```python
from build123d import *

# Parameters (mm, degrees)
SKETCH_1_R          = 12.5
EXTRUDE_1_DEPTH     = 27
CUT_EXTRUDE_START   = -37
CUT_EXTRUDE_1_DEPTH = 37
CUT_EXTRUDE_START_2 = 10
CUT_EXTRUDE_2_DEPTH = 43
SKETCH_4_W          = 14
SKETCH_4_H          = 25
CUT_EXTRUDE_3_DEPTH = 30
FILLET_1_R          = 4
SKETCH_7_R          = 4
SKETCH_5_R          = 4
CUT_EXTRUDE_4_DEPTH = 34
SKETCH_9_W          = 2.5
SKETCH_9_H          = 6
CUT_EXTRUDE_5_DEPTH = 34
SKETCH_10_R         = 1.5
CUT_EXTRUDE_6_DEPTH = 34
FILLET_3_R          = 1.5
SKETCH_11_R         = 2.5
EXTRUDE_2_DEPTH     = 14.5
SKETCH_12_R         = 2
EXTRUDE_3_DEPTH     = 10
FILLET_4_R          = 10


with BuildPart() as part:
    # 草图1 → 凸台-拉伸1 (new body)
    with BuildSketch(Plane(origin=(0, 0, 0), x_dir=(1, 0, 0), z_dir=(0, 1, 0))):
        with Locations(Location((0, 0, 0), (0, 0, 270))):
            Circle(SKETCH_1_R)
    extrude(amount=-EXTRUDE_1_DEPTH)

    # 草图2 → 切除-拉伸1 (cut)
    with BuildSketch(Plane(origin=(0, -27, 0), x_dir=(-1, 0, 0), z_dir=(0, -1, 0)).offset(CUT_EXTRUDE_START)):
        with BuildLine():
            Line((-10, 7.5), (10, 7.5))
            ThreePointArc((10, 7.5), (0, 12.5), (-10, 7.5))
        make_face()
        with BuildLine():
            Line((-10, -7.5), (10, -7.5))
            ThreePointArc((10, -7.5), (0, -12.5), (-10, -7.5))
        make_face()
    extrude(amount=CUT_EXTRUDE_1_DEPTH, mode=Mode.SUBTRACT)

    # 草图3 → 切除-拉伸2 (cut)
    with BuildSketch(Plane(origin=(0, 0, 0), x_dir=(1, 0, 0), z_dir=(0, 1, 0)).offset(CUT_EXTRUDE_START_2)):
        with BuildLine():
            Line((-12, 3.5), (-12, -3.5))
            ThreePointArc((-12, -3.5), (-12.5, 0), (-12, 3.5))
        make_face()
        with BuildLine():
            Line((12, 3.5), (12, -3.5))
            ThreePointArc((12, -3.5), (12.5, 0), (12, 3.5))
        make_face()
    extrude(amount=-CUT_EXTRUDE_2_DEPTH, mode=Mode.SUBTRACT)

    # 草图4 → 切除-拉伸3 (cut)
    with BuildSketch(Plane.XY.offset(7.5)):
        with Locations((0, -14.5)):
            Rectangle(SKETCH_4_W, SKETCH_4_H)
    extrude(amount=-CUT_EXTRUDE_3_DEPTH, mode=Mode.SUBTRACT)

    # 圆角1
    fillet_1_edges = [part.edges().sort_by_distance(p)[0] for p in [
        (-7, -2, 0),
        (7, -2, 0),
    ]]
    fillet(fillet_1_edges, radius=FILLET_1_R)

    # 草图7 → 放样2 section 0
    with BuildSketch(Plane(origin=(0, 0, 0), x_dir=(1, 0, 0), z_dir=(0, 1, 0))):
        Circle(SKETCH_7_R)
    # 草图5 → 放样2 section 1
    with BuildSketch(Plane(origin=(0, 1, 0), x_dir=(1, 0, 0), z_dir=(0, 1, 0))):
        Circle(SKETCH_5_R)
    loft()

    # 草图8 → 切除-拉伸4 (cut)
    with BuildSketch(Plane.ZY.offset(12)):
        with BuildLine():
            Line((-2, -27), (2, -27))
            Line((2, -27), (2, -20.464101615))
            ThreePointArc((2, -20.464101615), (0, -13), (-2, -20.464101615))
            Line((-2, -20.464101615), (-2, -27))
        make_face()
    extrude(amount=-CUT_EXTRUDE_4_DEPTH, mode=Mode.SUBTRACT)

    # 草图9 → 切除-拉伸5 (cut)
    with BuildSketch(Plane.ZY.offset(12)):
        with Locations((6.25, -24)):
            Rectangle(SKETCH_9_W, SKETCH_9_H)
        with Locations((-6.25, -24)):
            Rectangle(SKETCH_9_W, SKETCH_9_H)
    extrude(amount=-CUT_EXTRUDE_5_DEPTH, mode=Mode.SUBTRACT)

    # 草图10 → 切除-拉伸6 (cut)
    with BuildSketch(Plane.XY.offset(5)):
        with Locations(Location((-9.5, -24.5, 0), (0, 0, 270))):
            Circle(SKETCH_10_R)
        with Locations(Location((9.5, -24.5, 0), (0, 0, 270))):
            Circle(SKETCH_10_R)
    extrude(amount=-CUT_EXTRUDE_6_DEPTH, mode=Mode.SUBTRACT)

    # 圆角3
    fillet_3_edges = [part.edges().sort_by_distance(p)[0] for p in [
        (-12, -27, 2.75),
        (-12, -27, -2.75),
        (-7, -27, -3.5),
        (-7, -27, 3.5),
        (7, -27, -3.5),
        (7, -27, 3.5),
        (12, -27, 2.75),
        (12, -27, -2.75),
    ]]
    fillet(fillet_3_edges, radius=FILLET_3_R)

    # 草图11 → 凸台-拉伸2 (add)
    with BuildSketch(Plane(origin=(0, 1, 0), x_dir=(1, 0, 0), z_dir=(0, 1, 0))):
        with Locations(Location((0, 0, 0), (0, 0, 90))):
            Circle(SKETCH_11_R)
    extrude(amount=EXTRUDE_2_DEPTH)

    # 草图12 → 凸台-拉伸3 (add)
    with BuildSketch(Plane(origin=(0, 15.5, 0), x_dir=(1, 0, 0), z_dir=(0, 1, 0))):
        with Locations(Location((0, 0, 0), (0, 0, 270))):
            Circle(SKETCH_12_R)
    extrude(amount=EXTRUDE_3_DEPTH)

    # 圆角4
    # the kernel refuses this fillet: 10 mm, written as the material it takes off along each edge
    with BuildSketch(Plane(origin=(-9.535945694, -21, 7.5), x_dir=(0, 1, 0), z_dir=(1, 0, 0)), Plane(origin=(-26.535945694, -21, 7.5), x_dir=(0, 1, 0), z_dir=(1, 0, 0))) as fillet_4_piece_1:
        with BuildLine():
            CenterArc((6.614378278, -10), FILLET_4_R, 90, 41.409622109)
            Line((0, -2.5), (-0.132287566, -2.35))
            ThreePointArc((-0.132287566, -2.35), (-0.2, -1.25), (-0.2, 0))
            Line((-0.2, 0), (0, 0.2))
            Line((0, 0.2), (6.614378278, 0.2))
            Line((6.614378278, 0.2), (6.614378278, 0))
        make_face()
    extrude(amount=36.071891388, mode=Mode.SUBTRACT)
    with BuildSketch(Plane(origin=(-9.535945694, -21, -7.5), x_dir=(0, 0, 1), z_dir=(1, 0, 0))) as fillet_4_piece_2:
        with BuildLine():
            CenterArc((10, -6.614378278), FILLET_4_R, 138.590377891, 41.409622109)
            Line((0, -6.614378278), (-0.2, -6.614378278))
            Line((-0.2, -6.614378278), (-0.2, 0))
            Line((-0.2, 0), (0, 0.2))
            ThreePointArc((0, 0.2), (1.25, 0.2), (2.35, 0.132287566))
            Line((2.35, 0.132287566), (2.5, 0))
        make_face()
    extrude(amount=36.071891388, mode=Mode.SUBTRACT)
    with BuildSketch(Plane(origin=(-26.535945694, -21, -7.5), x_dir=(0, 1, 0), z_dir=(1, 0, 0))) as fillet_4_piece_3:
        with BuildLine():
            CenterArc((6.614378278, 10), FILLET_4_R, 228.590377891, 41.409622109)
            Line((0, 2.5), (-0.132287566, 2.35))
            ThreePointArc((-0.132287566, 2.35), (-0.2, 1.25), (-0.2, 0))
            Line((-0.2, 0), (0, -0.2))
            Line((0, -0.2), (6.614378278, -0.2))
            Line((6.614378278, -0.2), (6.614378278, 0))
        make_face()
    extrude(amount=36.071891388, mode=Mode.SUBTRACT)


solid = part.part
```
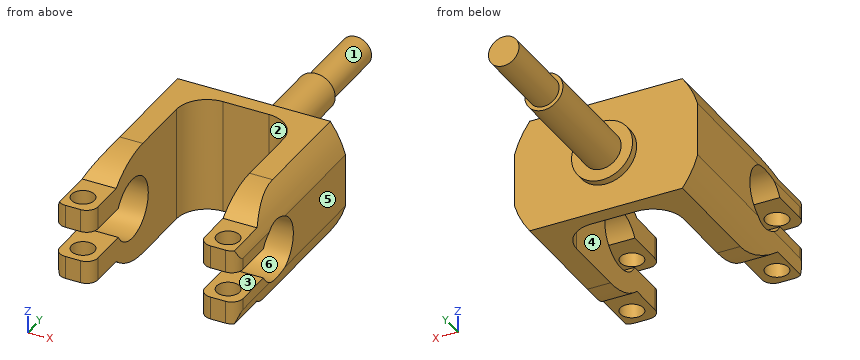
Design review of the part built by this model. Coordinates are the model's own, in mm. Face numbers are marked on the shaded views. A direction names the side the tool comes from. Coordinates: 2 decimals unless noted, no trailing zeros. Order: outer loops, then holes, each group sorted by start corner. A loop starts at its lowest first (then second) coordinate and runs counter-clockwise, first axis right, second up. Notation, with made-up numbers: (70.5, 53.25) - (74.5, 53.25) arc R12 cw to (74.5, 75.25) - close; hole circle Ø9 at (66, 82). An arc over 180 degrees is marked (long way). Answer in a Markdown table with one row per item.
(1) Clearance check with flat-ended pins moving along their axes: pin 1 (8 mm diameter, centred on x = -7.5, z = 2.5, fed in from +Y); pin 2 (1 mm diameter, centred on x = -7.5, y = -17.5, fed in from +Z); pin 3 (2.5 mm diameter, centred on x = 9.5, y = -25, fed in from +Z). State where each tip first meets the part, or that it passes through.
Checked values:
| item | result |
|---|---|
| pin 1 | y = 1 |
| pin 2 | z = 7.15 |
| pin 3 | z = 5 |
(2) Consider section A-A on x = 9.5. State the section outline as (y, z) points, plus the area to 3 significant figures.
Checked values:
| item | result |
|---|---|
| outline | (-27, -5) - (-26, -5) - (-26, -2) - (-27, -2) - close; (-27, 2) - (-26, 2) - (-26, 5) - (-27, 5) - close; (-23, -5) - (-21, -5) arc R10 ccw to (-14.39, -7.5) - (0, -7.5) - (0, 7.5) - (-14.39, 7.5) arc R10 ccw to (-21, 5) - (-23, 5) - (-23, 2) - (-20.46, 2) arc R4 cw (long way) to (-20.46, -2) - (-23, -2) - close |
| area | 272 mm^2 |
(3) Consider section D-D on z = 4.5. State the section outline as (x, y) points, plus the area to 3 significant figures.
Checked values:
| item | result |
|---|---|
| outline | (-11.66, -26.45) arc R1.5 ccw to (-10.5, -27) - (-8.5, -27) arc R1.5 ccw to (-7, -25.5) - (-7, -6) arc R4 cw to (-3, -2) - (3, -2) arc R4 cw to (7, -6) - (7, -25.5) arc R1.5 ccw to (8.5, -27) - (10.5, -27) arc R1.5 ccw to (11.66, -26.45) - (11.66, 0) - (-11.66, 0) - close; hole circle Ø3 at (-9.5, -24.5); hole circle Ø3 at (9.5, -24.5) |
| area | 271 mm^2 |
(4) Wall thickness on line 1 along X through (y, z) = (-24.5, 3.2); line 2 along Z through (x, y) = (8.5, -21); line 3 along X through (y, z) = (-24.5, -4.1): over which ranges is each line inside the solid? List them lowest first. Write a range as from..to.
Checked values:
| item | result |
|---|---|
| line 1 | -12..-11, -8..-7, 7..8, 11..12 |
| line 2 | -5..-2, 2..5 |
| line 3 | -11.81..-11, -8..-7, 7..8, 11..11.81 |
(5) Consider section B-B on y = -17. State the section outline as (x, z) points.
Checked values:
| item | result |
|---|---|
| outline | (-11.84, -4) arc R12.5 ccw to (-10.25, -7.15) - (-7, -7.15) - (-7, -4) - close; (-11.84, 4) - (-7, 4) - (-7, 7.15) - (-10.25, 7.15) arc R12.5 ccw to start; (7, -7.15) - (10.25, -7.15) arc R12.5 ccw to (11.84, -4) - (7, -4) - close; (7, 4) - (11.84, 4) arc R12.5 ccw to (10.25, 7.15) - (7, 7.15) - close |
(6) For the marked faces 1, 2 and 3, list the 3-axis set-ups (+Z, -Z, +X, -X, +Y, -Y) from which the entire face can be reached by the end or side of a thin tool; tool diameter is ignored.
Checked values:
| item | result |
|---|---|
| face 1 | +Y |
| face 2 | +Z, -Z, -Y |
| face 3 | +X, -X, -Y |
(7) Consider section C-C on x = 0. State the section outline as (y, z) points.
Checked values:
| item | result |
|---|---|
| outline | (-2, -7.5) - (0, -7.5) - (0, -4) - (1, -4) - (1, -2.5) - (15.5, -2.5) - (15.5, -2) - (25.5, -2) - (25.5, 2) - (15.5, 2) - (15.5, 2.5) - (1, 2.5) - (1, 4) - (0, 4) - (0, 7.5) - (-2, 7.5) - close |
(8) The part is to be moulded in two halves that separate along X. For the marked faces 4, 5 and 6, say which applies: released by +X, released by -X, zero draft, split by the parting line, or undercut.
Checked values:
| item | result |
|---|---|
| face 4 | undercut |
| face 5 | released by +X |
| face 6 | zero draft |
